```python
from build123d import *

# Parameters (mm, degrees)
SKETCH1_W                = 180
SKETCH1_H                = 90
BOSS_EXTRUDE1_DEPTH      = 8
SKETCH3_W                = 10
SKETCH3_H                = 10
CUT_EXTRUDE1_DEPTH       = 7
SKETCH4_W                = 25
SKETCH4_H                = 30
SKETCH4_W_2              = 45
SKETCH4_H_2              = 80
SKETCH4_W_3              = 46
SKETCH4_H_3              = 46
CUT_EXTRUDE2_DEPTH       = 4
SKETCH5_W                = 15.917599426
SKETCH5_H                = 22
SKETCH5_W_2              = 13.264666189
CUT_EXTRUDE3_DEPTH       = 101.940576578
CUT_EXTRUDE12_DEPTH      = 101.940576578
CUT_EXTRUDE12_DEPTH_BACK = 101.940576578
SKETCH6_W                = 42
SKETCH6_H                = 31


with BuildPart() as part:
    # Sketch1 → Boss-Extrude1 (new body)
    with BuildSketch(Plane.XY):
        Rectangle(SKETCH1_W, SKETCH1_H)
    extrude(amount=BOSS_EXTRUDE1_DEPTH)

    # Sketch3 → Cut-Extrude1 (cut)
    with BuildSketch(Plane(origin=(0, 0, 0), x_dir=(-1, 0, 0), z_dir=(0, 0, -1))):
        with Locations((-80, -35)):
            Rectangle(SKETCH3_W, SKETCH3_H)
        with Locations((-80, 35)):
            Rectangle(SKETCH3_W, SKETCH3_H)
        with Locations((80, 35)):
            Rectangle(SKETCH3_W, SKETCH3_H)
        with Locations((80, -35)):
            Rectangle(SKETCH3_W, SKETCH3_H)
    extrude(amount=-CUT_EXTRUDE1_DEPTH, mode=Mode.SUBTRACT)

    # Sketch4 → Cut-Extrude2 (cut)
    with BuildSketch(Plane(origin=(0, 0, 0), x_dir=(-1, 0, 0), z_dir=(0, 0, -1))):
        with Locations((52.5, 30)):
            Rectangle(SKETCH4_W, SKETCH4_H)
        with Locations((-27.5, 0)):
            Rectangle(SKETCH4_W_2, SKETCH4_H_2)
        with Locations((41, -12)):
            Rectangle(SKETCH4_W_3, SKETCH4_H_3)
    extrude(amount=-CUT_EXTRUDE2_DEPTH, mode=Mode.SUBTRACT)

    # Sketch5 → Cut-Extrude3 (cut, through all)
    with BuildSketch(Plane(origin=(0, 0, 0), x_dir=(-1, 0, 0), z_dir=(0, 0, -1))):
        with Locations((-82.041200287, 0)):
            Rectangle(SKETCH5_W, SKETCH5_H)
        with Locations((83.367666906, 0)):
            Rectangle(SKETCH5_W_2, SKETCH5_H)
    extrude(amount=-CUT_EXTRUDE3_DEPTH, mode=Mode.SUBTRACT)

    # Sketch6 → Cut-Extrude12 (cut, two sides: drawn at the far end of the back side and taken through both)
    with BuildSketch(Plane(origin=(0, 0, 0), x_dir=(-1, 0, 0), z_dir=(0, 0, -1)).offset(-CUT_EXTRUDE12_DEPTH_BACK)):
        with Locations((41, -9.5)):
            Rectangle(SKETCH6_W, SKETCH6_H)
    extrude(amount=CUT_EXTRUDE12_DEPTH + CUT_EXTRUDE12_DEPTH_BACK, mode=Mode.SUBTRACT)


solid = part.part
```
Geometry: final body of the model. Coordinates: model frame, mm. A direction names the side the tool comes from. Round coordinates to 2 decimals unless told otherwise and drop trailing zeros. Write each loop counter-clockwise with the first axis right and the second up, starting at its lowest first coordinate (ties: lowest second). Pieces come first, ordered by that corner, then holes. Notation, with made-up numbers: (-1.75, 5) -> (10.25, 5) arc R23 ccw to (10.25, 30) -> close; hole circle Ø7 at (-21.5, 31). An arc over 180 degrees is marked (long way). Return JSON: item names as keys, results as strings.
Q1. Section B-B on y = 1.5. Return the cut outline in (x, z), and give its area (3 significant figures).
From the geometry:
{"outline": "(-76.74, 0) -> (-64, 0) -> (-64, 4) -> (-62, 4) -> (-62, 8) -> (-76.74, 8) -> close; (-20, 4) -> (-18, 4) -> (-18, 0) -> (5, 0) -> (5, 4) -> (50, 4) -> (50, 0) -> (74.08, 0) -> (74.08, 8) -> (-20, 8) -> close", "area": "675 mm2"}
Q2. Section A-A on x = -60. Return the cut outline in (y, z).
From the geometry:
{"outline": "(-45, 0) -> (-35, 0) -> (-35, 4) -> (-25, 4) -> (-25, 8) -> (-45, 8) -> close; (6, 4) -> (11, 4) -> (11, 0) -> (15, 0) -> (15, 4) -> (45, 4) -> (45, 8) -> (6, 8) -> close"}
Q3. First-contact query: pin 1 Ø10 at (x, y) = (33, 11) entering from -Z; pin 2 Ø5 at (x, y) = (-81.5, -35.5) entering from -Z; pin 3 Ø2.5 at (y, z) = (3.5, 4.5) entering from +X. Flat tips, straight axial feed; report the tip coordinate or a pass-through.
From the geometry:
{"pin 1": "z = 4", "pin 2": "z = 7", "pin 3": "x = 74.08"}
Q4. Section D-D on y = 24.5. Return the cut outline in (x, z).
From the geometry:
{"outline": "(-90, 0) -> (-65, 0) -> (-65, 4) -> (-40, 4) -> (-40, 0) -> (5, 0) -> (5, 4) -> (50, 4) -> (50, 0) -> (90, 0) -> (90, 8) -> (-90, 8) -> close"}
Q5. Ray query, line 1 (X direction, y = 22.5, z = 1.25); line 2 (X direction, y = 33.5, z = 1.25); line 3 (X direction, y = 35, z = 5). Return the intervals inside material, ascending.
From the geometry:
{"line 1": "-90 to -65, -40 to 5, 50 to 90", "line 2": "-90 to -85, -75 to -65, -40 to 5, 50 to 75, 85 to 90", "line 3": "-90 to -85, -75 to 75, 85 to 90"}
Q6. Set-up query: faces 1 (the flat face through (-52, 30, 4)), 2 (the flat face through (74.082, 0, 4)), 3 (the flat face through (-62, -10, 6)), 4 (the flat face through (-75, 35, 3)), 5 (the flat face through (-76.735, 0, 4)). Return all of +Z, -Z, +X, -X, +Y, -Y with unobstructed straight access to the full face (end or side cutting, diameter ignored); none if empty.
From the geometry:
{"face 1": "-Z, +Y", "face 2": "+Z, -Z, +X", "face 3": "+Z, -Z", "face 4": "-Z", "face 5": "+Z, -Z, -X"}
Q7. Section C-C on z = 5.25. Give the number of separate pieces and of enclosed holes in the cut face, and give its area (3 significant figures).
From the geometry:
{"separate pieces": "1", "enclosed holes": "5", "area": "13,900 mm2"}
Q8. Mould query, pull axis Y, two halves, no side actions, for faces 6 (the flat face through (-1, 1, 8)), 7 (the flat face through (75, -35, 3)). Classes: +Y half, -Y half, draft (parallel to the pull), parting line (faces both ways), or undercut.
From the geometry:
{"face 6": "draft", "face 7": "undercut"}
